from build123d import *

# Parameters (mm, degrees)
F1_DEPTH = 40
F2_R     = 4.85
F3_DEPTH = 7.07
F4_R     = 4.85
F5_DEPTH = 7.07
F10_SIZE = 1


# Not quite as in the source:
# - a feature names something its author has since deleted; it is built from what else it names


with BuildPart() as f1:
    # F0 (on Right) → F1 (new body)
    with BuildSketch(Plane.YZ):
        with BuildLine():
            ThreePointArc((7.5, 5), (6.767766953, 6.767766953), (5, 7.5))
            Line((5, 7.5), (-5, 7.5))
            ThreePointArc((-5, 7.5), (-6.767766953, 6.767766953), (-7.5, 5))
            Line((-7.5, 5), (-7.5, -5))
            ThreePointArc((-7.5, -5), (-6.767766953, -6.767766953), (-5, -7.5))
            Line((-5, -7.5), (5, -7.5))
            ThreePointArc((5, -7.5), (6.767766953, -6.767766953), (7.5, -5))
            Line((7.5, -5), (7.5, 5))
        make_face()
    extrude(amount=F1_DEPTH)

    # F2 (on face) → F3 (cut)
    with BuildSketch(Plane.YZ.offset(40)):
        with Locations((0, -1.5)):
            Circle(F2_R)
    extrude(amount=-F3_DEPTH, mode=Mode.SUBTRACT)

    # F4 (on face) → F5 (cut)
    with BuildSketch(Plane.YZ):
        with Locations((0, -1.5)):
            Circle(F4_R)
    extrude(amount=F5_DEPTH, mode=Mode.SUBTRACT)

    # F6 (on Front) → F7 (revolve, cut)
    with BuildSketch(Plane.XZ):
        Polygon((32.93, -1.5), (32.93, 1), (10.5341016151, -1), (7.07, 1), (7.07, -1.5), align=None)
    revolve(axis=Axis((20, 0, -1.5), (1, 0, 0)), mode=Mode.SUBTRACT)

    # F8 (on Front) → F9 (revolve, cut)
    with BuildSketch(Plane.XZ):
        Polygon((9.57, 2.1126677044), (11.92, 2.1126677044), (14.42, 2.1126677044), (14.42, 9.1826677044), (9.57, 9.1826677044), align=None)
        Polygon((14.42, 2.1126677044), (11.92, 2.1126677044), (12.92, -0.8873322956), (14.42, -0.7533791963), align=None)
    revolve(axis=Axis((14.42, 0, 2.2679000954), (0, 0, -1)), mode=Mode.SUBTRACT)

    # F10
    f10_edges = [f1.edges().sort_by_distance(p)[0] for p in [
        (32.93, -4.85, -1.5),
        (7.07, -4.85, -1.5),
    ]]
    chamfer(f10_edges, length=F10_SIZE)


solid = f1.part
CAD build for the part. Positions are in the model's coordinates, mm. A direction names the side the tool comes from. Coordinates: 2 decimals unless noted, no trailing zeros. Loops run counter-clockwise (first coordinate to the right, second up) from the corner with the lowest first, then second, coordinate; pieces in that order, holes last. Notation, with made-up numbers: (87, 23.5) - (96, 23.5) arc R23 ccw to (96, 50.5) - close; hole circle Ø4 at (-21, 25). An arc over 180 degrees is marked (long way). Write item = value, one per line. Start each with the question number.
Q1. Flat gauge pins, fed straight in: pin 1 Ø6 at (y, z) = (0, -1.5) entering from -X; pin 2 Ø8 at (y, z) = (0, -1.5) entering from -X; pin 3 Ø5 at (y, z) = (1.5, -2) entering from +X. Where does each tip first touch, or does it go through?
Q2. Cut at B-B, the plane x = 37.5. List the corners of the cut face in (y, z), then the cut area to 3 significant figures.
Q3. Pull direction Z, two halves, no side cores. Call faces 4 (the flat face through (17, 1, 2.113)), 5 (the flat face through (20, 0, -7.5)), 6 (the flat face through (32.93, 3, -1)): pulls with the +Z half, pulls with the -Z half, needs draft (parallel to the pull), parting line crosses it, or undercut.
Q4. Cut at D-D, the plane x = 28. List the corners of the cut face in (y, z).
Q5. Cut at A-A, the plane y = 0. Give the number of separate pieces and of enclosed holes in the cut face, then the cut area to 3 significant figures.
Q6. Drill centre lines: L1, parallel to Z at x = 3, y = 0.25; L2, parallel to Y at x = 14.42, z = 4.25; L3, parallel to Z at x = 19, y = 0.5. Where is each one in solid material? Low to high.
Q7. Which spindle directions (+Z, -Z, +X, -X, +Y, -Y) get a long thin tool onto all of the face, cutting with end or side? Do faces 1 (the conical face through (21.575, -0.065, -2.985)), 2 (the conical face through (14.32, -0.85, -0.83)), 3 (the flat face through (7.07, 3, -1)). Say none if no direction does.
Q8. Cut at C-C, the plane z = 6.5. List the corners of the cut face in (x, y).
Computed:
q1.pin_1 = 7.07
q1.pin_2 = 6.92
q1.pin_3 = 33.16
q2.outline = (-7.5, -5) arc R2.5 ccw to (-5, -7.5) - (5, -7.5) arc R2.5 ccw to (7.5, -5) - (7.5, 5) arc R2.5 ccw to (5, 7.5) - (-5, 7.5) arc R2.5 ccw to (-7.5, 5) - close; hole circle Ø9.7 at (0, -1.5)
q2.area = 146 mm²
q3.face_4 = pulls with the +Z half
q3.face_5 = pulls with the -Z half
q3.face_6 = undercut
q4.outline = (-7.5, -5) arc R2.5 ccw to (-5, -7.5) - (5, -7.5) arc R2.5 ccw to (7.5, -5) - (7.5, 5) arc R2.5 ccw to (5, 7.5) - (-5, 7.5) arc R2.5 ccw to (-7.5, 5) - close; hole circle Ø4.12 at (0, -1.5)
q5.separate_pieces = 3
q5.enclosed_holes = 0
q5.area = 324 mm²
q6.L1 = -7.5 to -6.34, 3.34 to 7.5
q6.L2 = -7.5 to -4.85, 4.85 to 7.5
q6.L3 = -7.5 to -2.65, -0.35 to 2.11
q7.face_1 = +X
q7.face_2 = +Z
q7.face_3 = -X
q8.outline = (0, -7) - (40, -7) - (40, 7) - (0, 7) - close; hole circle Ø9.7 at (14.42, 0)
